```python
from build123d import *

# Parameters (mm, degrees)
CUT_EXTRUDE1_DEPTH = 0.75
FILLET1_R          = 0.125


with BuildPart() as part:
    # Sketch1 → Revolve1 (revolve)
    with BuildSketch(Plane(origin=(0, 0, 0), x_dir=(0, 0, -1), z_dir=(1, 0, 0))):
        with BuildLine():
            Line((0, 1.5), (-1.75, 1.5))
            ThreePointArc((-1.75, 1.5), (-2.334912942, 0.942930354), (-2.75, 0.25))
            Line((-2.75, 0.25), (-2.605662433, 0))
            Line((-2.605662433, 0), (-1.5, 0))
            Line((-1.5, 0), (-1.5, -8))
            Line((-1.5, -8), (0, -8))
            Line((0, -8), (0, 1.5))
        make_face()
    revolve(axis=Axis((0, -8, 0), (0, 1, 0)))

    # Sketch2 → Cut-Extrude1 (cut)
    with BuildSketch(Plane(origin=(0, 1.5, 0), x_dir=(1, 0, 0), z_dir=(0, 1, 0))):
        Polygon((0, 1.154700538), (-1, 0.577350269), (-1, -0.577350269), (0, -1.154700538), (1, -0.577350269), (1, 0.577350269), align=None)
    extrude(amount=-CUT_EXTRUDE1_DEPTH, mode=Mode.SUBTRACT)

    # Fillet1
    fillet1_edges = [part.edges().sort_by_distance(p)[0] for p in [
        (0.5, 1.5, -0.866025404),
        (-0.5, 1.5, -0.866025404),
        (-1, 1.5, 0),
        (-0.5, 1.5, 0.866025404),
        (0.5, 1.5, 0.866025404),
        (1, 1.5, 0),
        (0, 1.5, -1.75),
    ]]
    fillet(fillet1_edges, radius=FILLET1_R)


solid = part.part
```
The listing builds one solid part. Answer for the finished solid, in the listing's coordinates (mm). A direction names the side the tool comes from. Coordinates: 2 decimals unless noted, no trailing zeros. Loops run counter-clockwise (first coordinate to the right, second up) from the corner with the lowest first, then second, coordinate; pieces in that order, holes last. Notation, with made-up numbers: (66, 89) -> (90, 89) arc R25 ccw to (90, 124) -> close; hole circle Ø6 at (82, 47.5). An arc over 180 degrees is marked (long way). Return JSON: item names as keys, results as strings. Group by question number.
(1) Determine the mould class of faces 1 (the cylindrical face through (0.07, -4.06, -1.5)), 2 (the flat face through (0, 0.75, 0)), 3 (the flat face through (0, -8, 0)) for opening direction Z: released by +Z, released by -Z, zero draft, split by the parting line, or undercut.
(2) Which of the six approach directions +Z, -Z, +X, -X, +Y, -Y give full straight-line access (tool end or side, diameter ignored) to faces 4 (the flat face through (-1, 1.5, 1)), 5 (the flat face through (-2, 0, 0))?
(3) Given pin 1 Ø1 at (y, z) = (-2.5, 1) entering from +X; pin 2 Ø0.6 at (x, z) = (-0.5, 0) entering from +Y; pin 3 Ø0.5 at (y, z) = (1, -0.5) entering from -X, each flat-ended and moving along its own axis, determine where each tip first touches the part or whether it passes through.
(4) A cutting plane is placed at A-A on y = -0.5. Write down the section's boundary in (x, z), and give its area (3 significant figures).
(5) Find the intervals of material crossed by probe 1 along Y at (x, z) = (-0.3, -0.75); probe 2 along X at (y, z) = (1, 0.5); probe 3 along Y at (x, z) = (0.55, -1.6), in increasing order. Write a range as from..to.
The answers:
{
 "1": {"face 1": "split by the parting line", "face 2": "undercut", "face 3": "zero draft"},
 "2": {"face 4": "+Z, -Z, +X, -X, +Y", "face 5": "-Y"},
 "3": {"pin 1": "stops at x = 1.41", "pin 2": "stops at y = 0.75", "pin 3": "stops at x = -2.43"},
 "4": {"outline": "circle Ø3 at (0, 0)", "area": "7.07 mm^2"},
 "5": {"probe 1": "y = -8..0.75", "probe 2": "x = -2.23..-1, 1..2.23", "probe 3": "y = 0..1.5"}
}
